```python
from build123d import *

# Parameters (mm, degrees)
BOSS_EXTRUDE1_DEPTH = 10


with BuildPart() as part:
    # Sketch1 → Boss-Extrude1 (new body)
    with BuildSketch(Plane(origin=(0, 0, 0), x_dir=(1, 0, 0), z_dir=(0, 1, 0))):
        with BuildLine():
            Line((0, 0), (5, 0))
            Line((5, 0), (13.535533906, 6.464466094))
            Line((13.535533906, 6.464466094), (15, 10))
            Line((15, 10), (15, 65))
            ThreePointArc((15, 65), (13.708286934, 57.928932188), (10, 51.771243445))
            Line((10, 51.771243445), (10, 20))
            Line((10, 20), (10, 10))
            Line((10, 10), (5, 5))
            Line((5, 5), (0, 5))
            Line((0, 5), (0, 0))
        make_face()
    extrude(amount=BOSS_EXTRUDE1_DEPTH)


solid = part.part
```
Read the model definition and answer for the solid it produces. Units are mm, in the model's axes. A direction names the side the tool comes from. Round coordinates to 2 decimals unless told otherwise and drop trailing zeros. Write each loop counter-clockwise with the first axis right and the second up, starting at its lowest first coordinate (ties: lowest second). Pieces come first, ordered by that corner, then holes. Notation, with made-up numbers: (30.25, 43.5) - (71.25, 43.5) arc R16 ccw to (71.25, 69.5) - close; hole circle Ø1 at (10, 7.25). An arc over 180 degrees is marked (long way). One line per item, written item: value.
Q1. Find section B-B (x = 3.75). Determine the outline of the cut face in (y, z).
The answers:
outline: (0, -5) - (10, -5) - (10, 0) - (0, 0) - close
Q2. Which of the six approach directions +Z, -Z, +X, -X, +Y, -Y give full straight-line access (tool end or side, diameter ignored) to faces 1 (the flat face through (3, 5, -5)), 2 (the flat face through (14.26, 4.93, -8.21))?
The answers:
face 1: -Z, -X, +Y, -Y
face 2: +Z, +X, +Y, -Y
Q3. Find section A-A (y = 4.25). Determine the outline of the cut face in (x, z).
The answers:
outline: (0, -5) - (5, -5) - (10, -10) - (10, -51.77) arc R20 cw to (15, -65) - (15, -10) - (13.54, -6.46) - (5, 0) - (0, 0) - close
Q4. Straight lines are drawn through the part: line 1 (X direction, y = 9.5, z = -46); line 2 (Z direction, x = 1, y = 0.5); line 3 (Z direction, x = 11, y = 3.75). For each, find the intervals that lie inside material, in ascending order. Write a range as from..to.
The answers:
line 1: x = 10..15
line 2: z = -5..0
line 3: z = -53..-4.54
Q5. Each of these flat-tipped pins is pushed along its axis until it touches: P1, Ø1.5, axis at x = 3, y = 7.5, coming from the -Z side; P2, Ø1.5, axis at x = 5, y = 1, coming from the +Z side; P3, Ø5, axis at x = 3.5, y = 5.5, coming from the -Z side; P4, Ø1.5, axis at x = 10.5, y = 3, coming from the +Z side. Where does it stop, or does it pass through?
The answers:
P1: stops at z = -5
P2: stops at z = 0
P3: stops at z = -6
P4: stops at z = -3.6
Q6. Find section C-C (z = -43.5). Determine the outline of the cut face in (x, y), and give its area (3 significant figures).
The answers:
outline: (10, 0) - (15, 0) - (15, 10) - (10, 10) - close
area: 50.0 mm2
